from build123d import *

# Parameters (mm, degrees)
CROQUIS1_R              = 10.5
SALIENTE_EXTRUIR1_DEPTH = 8
CROQUIS5_R              = 3
CORTAR_EXTRUIR1_DEPTH   = 15


with BuildPart() as part:
    # Croquis1 → Saliente-Extruir1 (new body)
    with BuildSketch(Plane.XY):
        Circle(CROQUIS1_R)
    extrude(amount=SALIENTE_EXTRUIR1_DEPTH)

    # Croquis3 → Revolución1 (revolve)
    with BuildSketch(Plane(origin=(0, 0, 0), x_dir=(0, 0, -1), z_dir=(1, 0, 0))):
        with BuildLine():
            Line((-8, 10.5), (-10.428215768, 9.105809129))
            ThreePointArc((-10.428215768, 9.105809129), (-14.286975998, 5.260880841), (-15.7, 0))
            Line((-15.7, 0), (-8, 0))
            Line((-8, 0), (-8, 10.5))
        make_face()
    revolve(axis=Axis((0, 0, 8), (0, 0, 1)))

    # Croquis4 → Revolución2 (revolve)
    with BuildSketch(Plane(origin=(0, 0, 0), x_dir=(0, 0, -1), z_dir=(1, 0, 0))):
        with BuildLine():
            Line((0, 0), (0, 10.5))
            Line((0, 10.5), (0.623533648, 10.5))
            ThreePointArc((0.623533648, 10.5), (2.319891977, 10.168017325), (3.765956272, 9.221052632))
            ThreePointArc((3.765956272, 9.221052632), (7.765081748, 7.825826873), (11.4, 10))
            Line((11.4, 10), (16.3, 10))
            Line((16.3, 10), (16.3, 0))
            Line((16.3, 0), (0, 0))
        make_face()
    revolve(axis=Axis((0, 0, 0), (0, 0, -1)))

    # Croquis5 → Cortar-Extruir1 (cut)
    with BuildSketch(Plane(origin=(0, 0, -16.3), x_dir=(-1, 0, 0), z_dir=(0, 0, -1))):
        Circle(CROQUIS5_R)
    extrude(amount=-CORTAR_EXTRUIR1_DEPTH, mode=Mode.SUBTRACT)


solid = part.part
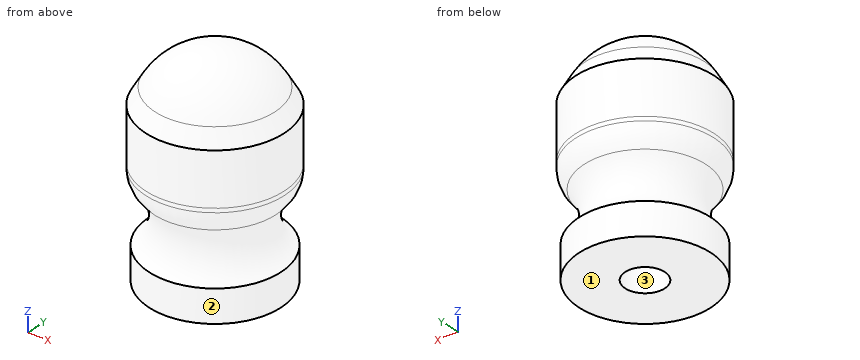
Geometry check sheet. Reference: the model listing, model coordinates, mm. Face numbers are marked on the shaded views. Coordinates: 2 decimals unless noted, no trailing zeros. Loops run counter-clockwise (first coordinate to the right, second up) from the corner with the lowest first, then second, coordinate; pieces in that order, holes last. Notation, with made-up numbers: (61, 54.5) - (112, 54.5) arc R19 cw to (112, 74.5) - close; hole circle Ø10 at (25.5, -29.75). An arc over 180 degrees is marked (long way). Use one line per item in the form item = value. Start each with the question number.
Item 1: Mould release check, pull along X, two halves, no side actions. Record for the marked faces 1, 2 and 3: +X half, -X half, draft (parallel to the pull), parting line (faces both ways), or undercut.
Item 2: Gauge pin test, flat ends, axial feed: pin 1 (3 mm diameter, centred on x = 5.5, z = 8.5, fed in from +Y); pin 2 (8 mm diameter, centred on x = -0.5, z = -10, fed in from +Y); pin 3 (12 mm diameter, centred on y = 0, z = 11, fed in from -X); pin 4 (1 mm diameter, centred on x = 0, y = -2, fed in from +Z). Record the tip position at first contact, or that the pin passes through.
Item 3: Section check A-A, the plane x = 0. Enter the section's corners in (y, z), and give its area (3 significant figures).
Item 4: Thickness scan on probe 1 along Y at (x, z) = (0, -11); probe 2 along X at (y, z) = (0, 0.5); probe 3 along Z at (x, y) = (1.5, 9.5). Record the ranges inside material, lowest first.
Computed:
q1.face_1 = draft
q1.face_2 = parting line
q1.face_3 = undercut
q2.pin_1 = 9.67
q2.pin_2 = 10
q2.pin_3 = -10.5
q2.pin_4 = 15.59
q3.outline = (-10.5, -0.62) arc R4.5 ccw to (-9.22, -3.77) arc R5 cw to (-10, -11.4) - (-10, -16.3) - (-3, -16.3) - (-3, -1.3) - (3, -1.3) - (3, -16.3) - (10, -16.3) - (10, -11.4) arc R5 cw to (9.22, -3.77) arc R4.5 ccw to (10.5, -0.62) - (10.5, 8) - (9.11, 10.43) arc R10.5 ccw to (-9.11, 10.43) - (-10.5, 8) - close
q3.area = 496 mm2
q4.probe_1 = -9.48 to -3, 3 to 9.48
q4.probe_2 = -10.5 to 10.5
q4.probe_3 = -16.3 to -11.11, -3.3 to 9.54
